The listing builds one solid part. Answer for the finished solid, in the listing's coordinates (mm). Face numbers are marked on the shaded views. Give positions to 0.01 mm unless a question says otherwise; leave off trailing zeros. Write each loop counter-clockwise with the first axis right and the second up, starting at its lowest first coordinate (ties: lowest second). Pieces come first, ordered by that corner, then holes. Notation, with made-up numbers: (-36.5, 8) -> (-31.5, 8) arc R22 ccw to (-31.5, 46) -> close; hole circle Ø9 at (15, -6.75). An arc over 180 degrees is marked (long way). Put each result on its own line as item: value. Start each with the question number.
1) Find the intervals of material crossed by line 1 along Y through (x, z) = (0, 4.75); line 2 along Y through (x, z) = (-3.75, 9.25); line 3 along Y through (x, z) = (8, 8), in increasing order. Write a range as from..to.
2) A cutting plane is placed at C-C (x = 0). Write down the section's boundary in (y, z).
3) A cutting plane is placed at A-A (z = 12). Write down the section's boundary in (x, y).
4) A cutting plane is placed at D-D (x = 8). Write down the section's boundary in (y, z), then the cut area to 3 significant figures.
5) For a pull along X with two mould halves and no side action, classify the marked faces 1, 2 and 3 as released by +X, released by -X, zero draft, split by the parting line, or undercut.
6) Flat-ended cylindrical pins translate along their axes: pin 1 Ø3 at (x, y) = (4.5, -25.5) entering from +Z; pin 2 Ø1 at (x, y) = (-5.5, -14.5) entering from +Z. Find the tip coordinate at first contact, or state that the pin passes through.
7) A cutting plane is placed at B-B (y = 0). Write down the section's boundary in (x, z), then the cut area to 3 significant figures.
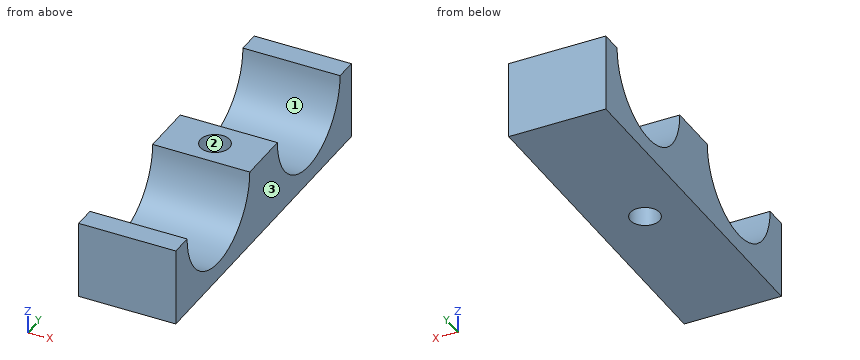
from build123d import *

# Parameters (mm, degrees)
SZKIC1_W                    = 20
SZKIC1_H                    = 70
DODANIE_WYCI_GNI_CIE1_DEPTH = 16
SZKIC2_R                    = 12.5
WYTNIJ_WYCI_GNI_CIE1_DEPTH  = 44.370496884
SZKIC3_R                    = 3
WYTNIJ_WYCI_GNI_CIE2_DEPTH  = 40.761790704


with BuildPart() as part:
    # Szkic1 → Dodanie-wyciągnięcie1 (new body)
    with BuildSketch(Plane.XY):
        Rectangle(SZKIC1_W, SZKIC1_H)
    extrude(amount=DODANIE_WYCI_GNI_CIE1_DEPTH)

    # Szkic2 → Wytnij-wyciągnięcie1 (cut, through all)
    with BuildSketch(Plane.ZY.offset(10)):
        with Locations((16, 18)):
            Circle(SZKIC2_R)
        with Locations((16, -18)):
            Circle(SZKIC2_R)
    extrude(amount=-WYTNIJ_WYCI_GNI_CIE1_DEPTH, mode=Mode.SUBTRACT)

    # Szkic3 → Wytnij-wyciągnięcie2 (cut, through all)
    with BuildSketch(Plane.XY.offset(16)):
        Circle(SZKIC3_R)
    extrude(amount=-WYTNIJ_WYCI_GNI_CIE2_DEPTH, mode=Mode.SUBTRACT)


solid = part.part
Reply:
1. line 1: y = -35..-23.45, -12.55..-3, 3..12.55, 23.45..35
1. line 2: y = -35..-28.52, -7.48..7.48, 28.52..35
1. line 3: y = -35..-27.6, -8.4..8.4, 27.6..35
2. outline: (-35, 0) -> (-3, 0) -> (-3, 16) -> (-5.5, 16) arc R12.5 cw to (-30.5, 16) -> (-35, 16) -> close; (3, 0) -> (35, 0) -> (35, 16) -> (30.5, 16) arc R12.5 cw to (5.5, 16) -> (3, 16) -> close
3. outline: (-10, -35) -> (10, -35) -> (10, -29.84) -> (-10, -29.84) -> close; (-10, -6.16) -> (10, -6.16) -> (10, 6.16) -> (-10, 6.16) -> close; (-10, 29.84) -> (10, 29.84) -> (10, 35) -> (-10, 35) -> close; hole circle Ø6 at (0, 0)
4. outline: (-35, 0) -> (35, 0) -> (35, 16) -> (30.5, 16) arc R12.5 cw to (5.5, 16) -> (-5.5, 16) arc R12.5 cw to (-30.5, 16) -> (-35, 16) -> close
4. area: 629 mm2
5. face 1: zero draft
5. face 2: undercut
5. face 3: released by +X
6. pin 1: stops at z = 7.33
6. pin 2: stops at z = 4.16
7. outline: (-10, 0) -> (-3, 0) -> (-3, 16) -> (-10, 16) -> close; (3, 0) -> (10, 0) -> (10, 16) -> (3, 16) -> close
7. area: 224 mm2
